For this review, take the finished solid that the model builds, in its own axes (mm). A direction names the side the tool comes from. Coordinates: 2 decimals unless noted, no trailing zeros. Order: outer loops, then holes, each group sorted by start corner. A loop starts at its lowest first (then second) coordinate and runs counter-clockwise, first axis right, second up. Notation, with made-up numbers: (82, -17) -> (113, -17) arc R25 ccw to (113, -4) -> close; hole circle Ø3 at (45, 70). An arc over 180 degrees is marked (long way). Answer as a JSON object with one key per item and string values. Group by question number.
1) Machinability: for faces 1 (the cylindrical face through (-3.56, 35.97, 1.83)), 2 (the cylindrical face through (2.142, 40.227, 2.676)), 3 (the flat face through (2.5, 17, 2)), which of the approach directions +Z, -Z, +X, -X, +Y, -Y give a long, thin tool a straight path to every point of the face, cutting with its end or side? Answer none if there is none.
2) Add section D-D, the plane x = -8.25. Write out the cut boundary in (y, z), then the cut area to 3 significant figures.
3) Wall thickness on L1, parallel to Y at x = -0.75, z = 3.35; L2, parallel to Y at x = 0, z = 1; L3, parallel to Y at x = 7.75, z = 0.75: over which ranges is each line inside the solid? List them lowest first.
4) Add section A-A, the plane x = -13.5. Write out the cut boundary in (y, z).
5) Draft analysis for pull direction X (two halves, no side actions). For faces 4 (the flat face through (4, 36, 1.725)), 5 (the flat face through (-5, 21, 2)), 6 (the flat face through (-2, 15, 3.6)), 7 (the cylindrical face through (4.8, -1.4, 1.8)), state which applies: +X half, -X half, draft (parallel to the pull), parting line (faces both ways), or undercut.
6) Add section B-B, the plane y = 24. Write out the cut boundary in (x, z), then the cut area to 3 significant figures.
7) Add section C-C, the plane z = 2.7. Write out the cut boundary in (x, y).
8) For pin 1 (1 mm diameter, centred on x = 1, z = 1, fed in from -Y); pin 2 (2.5 mm diameter, centred on x = 2.5, y = 37.5, fed in from +Z); pin 3 (1.5 mm diameter, centred on x = 7, z = 0.5, fed in from -Y); pin 4 (1 mm diameter, centred on x = -3.5, z = 0.5, fed in from +Y), all flat-tipped, find the tip position at first contact; note any pin that passes through.
from build123d import *

# Parameters (mm, degrees)
SKETCH1_R           = 1.6
BOSS_EXTRUDE1_DEPTH = 3.6
SKETCH2_R           = 0.75
CUT_EXTRUDE1_DEPTH  = 4.6
SKETCH4_R           = 2.75
CUT_EXTRUDE3_DEPTH  = 1.875


with BuildPart() as part:
    # Sketch1 → Boss-Extrude1 (new body)
    with BuildSketch(Plane.XY):
        with BuildLine():
            Line((-5, 37.5), (-5, 3.117408991))
            Line((-5, 3.117408991), (-15.45246273, -4.737424277))
            ThreePointArc((-15.45246273, -4.737424277), (-16.30801025, -8.97190619), (-12.202106424, -10.31516804))
            Line((-12.202106424, -10.31516804), (0, -5))
            ThreePointArc((0, -5), (4.829629131, -1.294095226), (2.5, 4.330127019))
            Line((2.5, 4.330127019), (2.5, 30))
            ThreePointArc((2.5, 30), (7.803300859, 42.803300859), (-5, 37.5))
        make_face()
        Circle(SKETCH1_R, mode=Mode.SUBTRACT)
        with Locations((-13.5, -7.335575406)):
            Circle(SKETCH1_R, mode=Mode.SUBTRACT)
        with Locations((2.5, 37.5)):
            Circle(SKETCH1_R, mode=Mode.SUBTRACT)
    extrude(amount=BOSS_EXTRUDE1_DEPTH)

    # Sketch2 → Cut-Extrude1 (cut, through all)
    with BuildSketch(Plane.XY.offset(3.6)):
        with Locations((7.668309414, 35.618889212)):
            Circle(SKETCH2_R)
        with BuildLine():
            ThreePointArc((-0.858757211, 40.858757211), (-0.858757211, 41.919417382), (-1.919417382, 41.919417382))
            ThreePointArc((-1.919417382, 41.919417382), (-3.537036414, 35.882380968), (0.882380968, 31.462963586))
            ThreePointArc((0.882380968, 31.462963586), (1.800939622, 31.993293672), (1.270609536, 32.911852325))
            ThreePointArc((1.270609536, 32.911852325), (-2.088147675, 36.270609536), (-0.858757211, 40.858757211))
        make_face()
    extrude(amount=-CUT_EXTRUDE1_DEPTH, mode=Mode.SUBTRACT)

    # Sketch4 → Cut-Extrude3 (cut)
    with BuildSketch(Plane.XY.offset(3.6)):
        with Locations((2.5, 37.5)):
            Circle(SKETCH4_R)
    extrude(amount=-CUT_EXTRUDE3_DEPTH, mode=Mode.SUBTRACT)


solid = part.part
Output values:
{
 "1": {"face 1": "+Z, -Z", "face 2": "+Z", "face 3": "+Z, -Z, +X"},
 "2": {"outline": "(-8.59, 0) -> (0.68, 0) -> (0.68, 3.6) -> (-8.59, 3.6) -> close", "area": "33.4 mm²"},
 "3": {"L1": "y = -5.33 to -1.41, 1.41 to 32.16, 34.04 to 41, 41.78 to 44.26", "L2": "y = -5 to -1.6, 1.6 to 31.77, 33.46 to 44.57", "L3": "y = 32.14 to 34.87, 36.36 to 42.86"},
 "4": {"outline": "(-10.59, 0) -> (-8.94, 0) -> (-8.94, 3.6) -> (-10.59, 3.6) -> close; (-5.74, 0) -> (-3.27, 0) -> (-3.27, 3.6) -> (-5.74, 3.6) -> close"},
 "5": {"face 4": "undercut", "face 5": "-X half", "face 6": "draft", "face 7": "+X half"},
 "6": {"outline": "(-5, 0) -> (2.5, 0) -> (2.5, 3.6) -> (-5, 3.6) -> close", "area": "27.0 mm²"},
 "7": {"outline": "(-15.45, -4.74) arc R3.25 ccw to (-12.2, -10.32) -> (0, -5) arc R5 ccw to (2.5, 4.33) -> (2.5, 30) arc R7.5 ccw (long way) to (-5, 37.5) -> (-5, 3.12) -> close; hole circle Ø3.2 at (-13.5, -7.34); hole (-1.92, 41.92) arc R6.25 ccw to (0.88, 31.46) arc R0.75 ccw to (1.27, 32.91) arc R4.75 cw to (-0.86, 40.86) arc R0.75 ccw to start; hole circle Ø3.2 at (0, 0); hole circle Ø5.5 at (2.5, 37.5); hole circle Ø1.5 at (7.67, 35.62)"},
 "8": {"pin 1": "stops at y = -4.97", "pin 2": "passes through", "pin 3": "stops at y = 31", "pin 4": "stops at y = 42.6"}
}
